Autodesk Inventor part; units mm, degrees
ref_plane "YZ Plane" through (0, 0, 0) normal (1, 0, 0) x (0, 1, 0)
ref_plane "XZ Plane" through (0, 0, 0) normal (0, 1, 0) x (-1, 0, 0)
ref_plane "XY Plane" through (0, 0, 0) normal (0, 0, 1) x (1, 0, 0)
sketch "Sketch1" plane through (0, 0, 0) normal (0, 0, 1) x (1, 0, 0)
  line L0 (0, 0) -> (-203.2, 0)
  line L1 (-203.2, 0) -> (-203.2, 86.36)
  line L2 (-203.2, 86.36) -> (0, 86.36)
  line L3 (0, 86.36) -> (0, 0)
  dimension "d0" = 203.2
  dimension "d1" = 86.36
extrude "Extrusion1" add sketch "Sketch1" along normal blind 0.254
sketch "Sketch2" plane through (0, 0, 0.254) normal (0, 0, 1) x (1, 0, 0)
  line L0 (-203.2, 0) -> (0, 0)
  line L1 (0, 0) -> (-0.254, 0)
  line L2 (-0.254, 0) -> (-0.254, 86.36)
  line L3 (-0.254, 86.36) -> (0, 86.36)
  line L4 (0, 86.36) -> (0, 0)
  dimension "d4" = 0.254
extrude "Extrusion2" add sketch "Sketch2" along normal blind 8.001
sketch "Sketch3" plane through (0, 0, 0) normal (1, 0, 0) x (0, 0, -1)
  point P0 (0, 0)
sketch "Sketch4" plane through (0, 0, 0.254) normal (0, 0, 1) x (1, 0, 0)
  line L0 (0, 0) -> (-203.2, 0)
  line L1 (-203.2, 86.36) -> (0, 86.36)
  line L2 (-35.56, 0) -> (-35.306, 0)
  line L3 (-35.306, 0) -> (-35.306, 86.36)
  line L4 (-35.306, 86.36) -> (-35.56, 86.36)
  line L5 (-35.56, 86.36) -> (-35.56, 0)
  dimension "d7" = 0.254
extrude "Extrusion3" add sketch "Sketch4" along normal blind 8.001
sketch "Sketch5" plane through (0, 0, 0.254) normal (0, 0, 1) x (1, 0, 0)
  line L0 (0, 0) -> (-203.2, 0)
  line L1 (-203.2, 86.36) -> (0, 86.36)
  line L2 (-71.12, 0) -> (-70.866, 0)
  line L3 (-70.866, 0) -> (-70.866, 86.36)
  line L4 (-70.866, 86.36) -> (-71.12, 86.36)
  line L5 (-71.12, 86.36) -> (-71.12, 0)
  line L6 (-106.68, 0) -> (-106.426, 0)
  line L7 (-106.426, 0) -> (-106.426, 86.36)
  line L8 (-106.426, 86.36) -> (-106.68, 86.36)
  line L9 (-106.68, 86.36) -> (-106.68, 0)
  line L10 (-142.24, 0) -> (-141.986, 0)
  line L11 (-141.986, 0) -> (-141.986, 86.36)
  line L12 (-141.986, 86.36) -> (-142.24, 86.36)
  line L13 (-142.24, 86.36) -> (-142.24, 0)
  line L14 (-177.8, 0) -> (-177.546, 0)
  line L15 (-177.546, 0) -> (-177.546, 86.36)
  line L16 (-177.546, 86.36) -> (-177.8, 86.36)
  line L17 (-177.8, 86.36) -> (-177.8, 0)
  dimension "d10" = 0.254
  dimension "d11" = 0.254
  dimension "d12" = 0.254
  dimension "d13" = 0.254
extrude "Extrusion4" add sketch "Sketch5" along normal blind 8.001 contours L0 L5 L1 L3
sketch "Sketch6" plane through (0, 0, 0.254) normal (0, 0, 1) x (1, 0, 0)
  line L0 (0, 0) -> (-203.2, 0)
  line L1 (-203.2, 86.36) -> (0, 86.36)
  line L2 (-106.68, 0) -> (-106.426, 0)
  line L3 (-106.426, 0) -> (-106.426, 86.36)
  line L4 (-106.426, 86.36) -> (-106.68, 86.36)
  line L5 (-106.68, 86.36) -> (-106.68, 0)
  dimension "d16" = 0.254
extrude "Extrusion5" add sketch "Sketch6" along normal blind 8.001
sketch "Sketch7" plane through (0, 0, 0.254) normal (0, 0, 1) x (1, 0, 0)
  line L0 (-203.2, 0) -> (-106.68, 0)
  line L1 (-106.68, 86.36) -> (-203.2, 86.36)
  line L2 (-142.24, 0) -> (-141.986, 0)
  line L3 (-141.986, 0) -> (-141.986, 86.36)
  line L4 (-141.986, 86.36) -> (-142.24, 86.36)
  line L5 (-142.24, 86.36) -> (-142.24, 0)
  point P0 (0, 0)
  dimension "d19" = 0.254
extrude "Extrusion6" add sketch "Sketch7" along normal blind 8.001
sketch "Sketch8" plane through (0, 0, 0.254) normal (0, 0, 1) x (1, 0, 0)
  line L0 (0, 0) -> (-203.2, 0)
  line L1 (-203.2, 86.36) -> (0, 86.36)
  line L2 (-177.8, 0) -> (-177.546, 0)
  line L3 (-177.546, 0) -> (-177.546, 86.36)
  line L4 (-177.546, 86.36) -> (-177.8, 86.36)
  line L5 (-177.8, 86.36) -> (-177.8, 0)
  dimension "d22" = 0.254
extrude "Extrusion7" add sketch "Sketch8" along normal blind 8.001
properties part number "ModuleHolder"
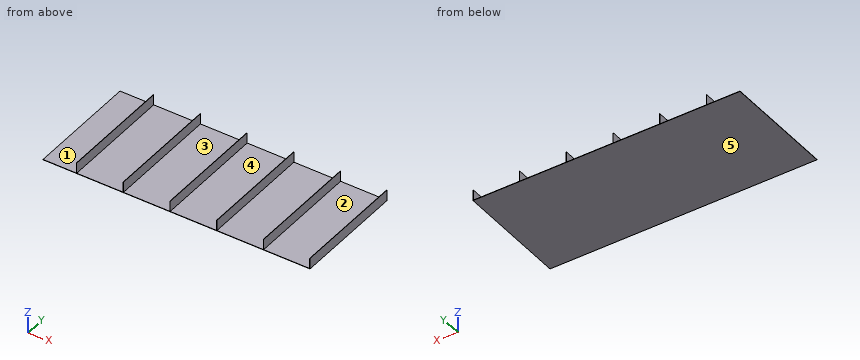
Read the model definition and answer for the solid it produces. Units are mm, in the model's axes. Face numbers are marked on the shaded views. A direction names the side the tool comes from. Coordinates: 2 decimals unless noted, no trailing zeros. Loops run counter-clockwise (first coordinate to the right, second up) from the corner with the lowest first, then second, coordinate; pieces in that order, holes last. Notation, with made-up numbers: (58.25, 44.25) -> (93.25, 44.25) arc R18 cw to (93.25, 48.25) -> close; hole circle Ø2 at (89, 51). An arc over 180 degrees is marked (long way). Write item = value, one per line. Start each with the question number.
1) Given P1, Ø2.5, axis at y = 39, z = 2.5, coming from the +X side; P2, Ø1.5, axis at x = -66, z = 3, coming from the +Y side; P3, Ø2, axis at x = -93, y = 76.5, coming from the +Z side; P4, Ø4, axis at y = 24.5, z = 5.5, coming from the -X side, each flat-ended and moving along its own axis, determine where each tip first touches the part or whether it passes through.
2) For the marked faces 4 and 5, determine the directions among +Z, -Z, +X, -X, +Y, -Y from which every point of the face is accessible in a straight line to the end or side of a thin tool.
3) The mould has two halves that part along X. Classify the marked faces 1, 2 and 3: pulls with the +X half, pulls with the -X half, needs draft (parallel to the pull), parting line crosses it, or undercut.
4) Find the intervals of material crossed by L1, parallel to X at y = 23, z = 4.75; L2, parallel to Z at x = -54, y = 50, in increasing order. Write a range as from..to.
5) The part is cut by section C-C, the plane x = -90.5. Determine the outline of the cut face in (y, z), plus the area to 3 significant figures.
6) The part is cut by section B-B, the plane y = 69.5. Determine the outline of the cut face in (x, z) (3 decimals), plus the area to 3 significant figures.
7) The part is cut by section A-A, the plane z = 2. Determine the outline of the cut face in (x, y).
Result:
q1.P1 = 0
q1.P2 = through
q1.P3 = 0.25
q1.P4 = -177.8
q2.face_4 = +Z, +Y, -Y
q2.face_5 = -Z, +X, -X, +Y, -Y
q3.face_1 = needs draft
q3.face_2 = undercut
q3.face_3 = undercut
q4.L1 = -177.8..-177.55, -142.24..-141.99, -106.68..-106.43, -71.12..-70.87, -35.56..-35.31, -0.25..0
q4.L2 = 0..0.25
q5.outline = (0, 0) -> (86.36, 0) -> (86.36, 0.25) -> (0, 0.25) -> close
q5.area = 21.9 mm²
q6.outline = (-203.2, 0) -> (0, 0) -> (0, 8.255) -> (-0.254, 8.255) -> (-0.254, 0.254) -> (-35.306, 0.254) -> (-35.306, 8.255) -> (-35.56, 8.255) -> (-35.56, 0.254) -> (-70.866, 0.254) -> (-70.866, 8.255) -> (-71.12, 8.255) -> (-71.12, 0.254) -> (-106.426, 0.254) -> (-106.426, 8.255) -> (-106.68, 8.255) -> (-106.68, 0.254) -> (-141.986, 0.254) -> (-141.986, 8.255) -> (-142.24, 8.255) -> (-142.24, 0.254) -> (-177.546, 0.254) -> (-177.546, 8.255) -> (-177.8, 8.255) -> (-177.8, 0.254) -> (-203.2, 0.254) -> close
q6.area = 63.8 mm²
q7.outline = (-177.8, 0) -> (-177.55, 0) -> (-177.55, 86.36) -> (-177.8, 86.36) -> close; (-142.24, 0) -> (-141.99, 0) -> (-141.99, 86.36) -> (-142.24, 86.36) -> close; (-106.68, 0) -> (-106.43, 0) -> (-106.43, 86.36) -> (-106.68, 86.36) -> close; (-71.12, 0) -> (-70.87, 0) -> (-70.87, 86.36) -> (-71.12, 86.36) -> close; (-35.56, 0) -> (-35.31, 0) -> (-35.31, 86.36) -> (-35.56, 86.36) -> close; (-0.25, 0) -> (0, 0) -> (0, 86.36) -> (-0.25, 86.36) -> close
